Input: part model. Units: mm. Frame: model coordinates. A direction names the side the tool comes from. Give positions to 0.01 mm unless a question says otherwise; leave off trailing zeros. Loops run counter-clockwise (first coordinate to the right, second up) from the corner with the lowest first, then second, coordinate; pieces in that order, holes last. Notation, with made-up numbers: (6.5, 15) -> (57.5, 15) arc R22 cw to (57.5, 41) -> close; hole circle Ø7 at (55, 73). An arc over 180 degrees is marked (long way). Use CSV: the item, a comma, the result in double quotes.
Autodesk Inventor part; units mm, degrees
ref_plane "YZ Plane" through (0, 0, 0) normal (1, 0, 0) x (0, 1, 0)
ref_plane "XZ Plane" through (0, 0, 0) normal (0, 1, 0) x (-1, 0, 0)
ref_plane "XY Plane" through (0, 0, 0) normal (0, 0, 1) x (1, 0, 0)
sketch "Sketch1" plane through (0, 0, 0) normal (0, 1, 0) x (-1, 0, 0)
  line L0 (-8.3746, 16.5585) -> (42.4254, 16.5585)
  line L1 (42.4254, 16.5585) -> (42.4254, 14.0185)
  line L2 (42.4254, 14.0185) -> (33.5354, 14.0185)
  line L3 (33.5354, 14.0185) -> (33.5354, -11.3815)
  line L4 (33.5354, -11.3815) -> (42.4254, -11.3815)
  line L5 (42.4254, -11.3815) -> (42.4254, -13.9215)
  line L6 (42.4254, -13.9215) -> (-8.3746, -13.9215)
  line L7 (-8.3746, 16.5585) -> (-8.3746, 14.0185)
  line L8 (-8.3746, 14.0185) -> (23.3754, 14.0185)
  line L9 (23.3754, 14.0185) -> (23.3754, -11.3815)
  line L10 (23.3754, -11.3815) -> (-8.3746, -11.3815)
  line L11 (-8.3746, -11.3815) -> (-8.3746, -13.9215)
  point P0 (0, 0)
  dimension "d0" = 30.48
  dimension "d1" = 2.54
  dimension "d2" = 2.54
  dimension "d4" = 2.54
  dimension "d5" = 2.54
  dimension "d6" = 8.89
  dimension "d7" = 50.8
  dimension "d8" = 31.75
extrude "Extrusion1" add sketch "Sketch1" along normal blind 25.4
sketch "Sketch4" plane through (8.3746, 0, -13.9215) normal (0, 0, -1) x (-1, 0, 0)
  line L0 (50.8, 0) -> (0, 0)
  line L1 (50.8, 0) -> (50.8, 25.4)
  line L2 (0, 25.4) -> (50.8, 25.4)
  line L3 (50.8, 25.4) -> (41.91, 25.4)
  line L4 (41.91, 25.4) -> (41.91, 0)
  line L5 (41.91, 0) -> (50.8, 0)
  line L6 (50.8, 0) -> (50.8, 25.4)
  point P0 (8.3746, 0)
  dimension "d56" = 8.89
extrude "Extrusion3" add sketch "Sketch4" along normal blind 11.43
sketch "Sketch5" plane through (-42.4254, 0, 16.5585) normal (0, 0, 1) x (1, 0, 0)
  line L0 (50.8, 0) -> (50.8, 25.4)
  line L1 (50.8, 0) -> (0, 0)
  point P0 (40.64, 12.7)
  dimension "d11" = 10.16
  dimension "d12" = 12.7
hole "Hole1" at (-1.7854, 12.7, 16.5585) direction (0, 0, -1) diameter 9.779 end through all
sketch "Sketch6" plane through (-42.4254, 0, 16.5585) normal (0, 0, 1) x (1, 0, 0)
  line L0 (0, 0) -> (0, 25.4)
  line L1 (50.8, 0) -> (0, 0)
  point P0 (4, 4)
  dimension "d20" = 4
  dimension "d21" = 4
hole "Hole2" at (-38.4254, 4, 16.5585) direction (0, 0, -1) diameter 4.5 end through all
sketch "Sketch2" plane through (-42.4254, 0, 16.5585) normal (0, 0, 1) x (1, 0, 0)
  circle A0 centre (40.64, 12.7) radius 4.8895
  line L0 (40.64, 22.225) -> (40.64, 3.175) construction
  circle A1 centre (40.64, 12.7) radius 4.8895 construction
  line L1 (40.64, 12.7) -> (33.9048, 19.4352) construction
  line L2 (40.64, 12.7) -> (33.9048, 5.9648) construction
  line L3 (40.64, 12.7) -> (47.3752, 5.9648) construction
  line L4 (40.64, 12.7) -> (47.3752, 19.4352) construction
  point P0 (42.4254, 0)
  dimension "d29" = 9.525
  dimension "d30" = 0
  dimension "d33" = 360
  dimension "d60" = 45
  dimension "d63" = 360
hole "Hole3" at (-1.7854, 3.175, 16.5585) at (-1.7854, 22.225, 16.5585) at (-8.5206, 5.9648, 16.5585) at (-8.5206, 19.4352, 16.5585) at (4.9498, 19.4352, 16.5585) at (4.9498, 5.9648, 16.5585) direction (0, 0, -1) diameter 2.794 end through all
fillet "Fillet2" radius 3.175 8 edges at (-42.4254, 0, -18.3665) (-42.4254, 0, 15.2885) (-23.3754, 12.7, 14.0185) (-23.3754, 12.7, -11.3815) (8.3746, 0, -12.6515) (8.3746, 25.4, -12.6515) (8.3746, 25.4, 15.2885) (8.3746, 0, 15.2885)
hole "Hole4" at (-33.5354, 22.1488, 1.9535) direction (1, 0, 0) diameter 3.81 end through all
sketch "Sketch7" plane through (8.3746, 0, -25.3515) normal (0, 0, -1) x (-1, 0, 0)
  circle A0 centre (46.355, 19.1807) radius 1.524
  circle A1 centre (46.355, 12.5767) radius 1.524
  line L0 (50.8, 3.175) -> (50.8, 25.4) construction
  line L1 (41.91, 25.4) -> (41.91, 0) construction
  line L2 (50.8, 25.4) -> (41.91, 25.4) construction
  point P0 (8.3746, 0)
  dimension "d65" = 3.048
  dimension "d66" = 3.048
  dimension "d67" = 6.604
  dimension "d68" = 8.89
  dimension "d69" = 4.445
  dimension "d70" = 4.445
  dimension "d71" = 6.2193
extrude "Extrusion4" cut sketch "Sketch7" against normal up to surface (13.97 mm away)
equation "\"d2\" = d1"
equation "\"d4\" = d1"
equation "\"d5\" = d1"
equation "\"d69\" = 0.5 * d68"
equation "\"d70\" = 0.5 * d68"
properties part number "Odometry_Holder-01"
1) Section query B-B (x = -4.5). Return loops of the section in (y, z).
From the geometry:
outline,"(0, -13.92) -> (8.63, -13.92) -> (8.63, -11.38) -> (0, -11.38) -> close; (0, 14.02) -> (8.63, 14.02) -> (8.63, 16.56) -> (0, 16.56) -> close; (16.77, -13.92) -> (25.4, -13.92) -> (25.4, -11.38) -> (16.77, -11.38) -> close; (16.77, 14.02) -> (25.4, 14.02) -> (25.4, 16.56) -> (16.77, 16.56) -> close"
2) Contact query for flat-ended pins moving along their axis: pin 1 (1 mm diameter, centred on y = 15.5, z = 3, fed in from +X); pin 2 (3 mm diameter, centred on y = 22.15, z = 1.95, fed in from +X); pin 3 (8 mm diameter, centred on x = 2, y = 20, fed in from -Z); pin 4 (7.5 mm diameter, centred on y = 8, z = 6, fed in from -X). Output: stop coordinate, or through.
From the geometry:
pin 1,"stops at x = -23.38"
pin 2,"passes through"
pin 3,"stops at z = -13.92"
pin 4,"stops at x = -33.54"
3) Mould query, pull axis Z, two halves, no side actions, for faces 1 (the cylindrical face through (4.006, 6.994, 15.271)), 2 (the flat face through (-36, 13, -25.352)), 3 (the cylindrical face through (-22.47, 12.878, 13.064)). Classes: pulls with the +Z half, pulls with the -Z half, needs draft (parallel to the pull), parting line crosses it, or undercut.
From the geometry:
face 1,"needs draft"
face 2,"pulls with the -Z half"
face 3,"undercut"
4) Reachability of faces 4 (the cylindrical face through (-9.699, 18.684, 15.271)), 5 (the cylindrical face through (-36.77, 11.65, -18.46)), 6 (the flat face through (-33.535, 13, 1)), 7 (the cylindrical face through (-22.421, 12.878, -10.476)) from +Z, -Z, +X, -X, +Y, -Y: full face, straight path, thin tool, end or side. Return the list, or none.
From the geometry:
face 4,"+Z, -Z"
face 5,"-Z"
face 6,"-X, +Y, -Y"
face 7,"+X, +Y, -Y"
5) Ray query, line 1 (Z direction, x = -17.5, y = 24); line 2 (Z direction, x = -38, y = 9.75); line 3 (X direction, y = 19.5, z = -6.5). Return the intervals inside material, ascending.
From the geometry:
line 1,"z = -13.92 to -11.38, 14.02 to 16.56"
line 2,"z = -25.35 to -11.38, 14.02 to 16.56"
line 3,"x = -33.54 to -23.38"
6) Section query D-D (x = -37.5). Return loops of the section in (y, z).
From the geometry:
outline,"(0, -25.35) -> (1.95, -25.35) -> (1.95, -11.38) -> (0, -11.38) -> close; (0, 14.02) -> (1.95, 14.02) -> (1.95, 16.56) -> (0, 16.56) -> close; (6.05, -25.35) -> (11.13, -25.35) -> (11.13, -11.38) -> (6.05, -11.38) -> close; (6.05, 14.02) -> (25.4, 14.02) -> (25.4, 16.56) -> (6.05, 16.56) -> close; (14.02, -25.35) -> (17.73, -25.35) -> (17.73, -11.38) -> (14.02, -11.38) -> close; (20.63, -25.35) -> (25.4, -25.35) -> (25.4, -11.38) -> (20.63, -11.38) -> close"
7) Section query A-A (y = 14.75). Give the number of separate pieces and of enclosed holes in the cut face, then the cut area to 3 significant figures.
From the geometry:
separate pieces,"3"
enclosed holes,"0"
area,"577 mm^2"
